Part model, mm, in its own coordinate system. A direction names the side the tool comes from. Give positions to 0.01 mm unless a question says otherwise; leave off trailing zeros. Order: outer loops, then holes, each group sorted by start corner. A loop starts at its lowest first (then second) coordinate and runs counter-clockwise, first axis right, second up. Notation, with made-up numbers: M 15,-21 L 57,-21 A19 cw 57,-12 Z; hole C 44.5,58.25 d6. An arc over 180 degrees is marked long. Answer as a JSON object with one key per item and string values.
from build123d import *

# Parameters (mm, degrees)
SKETCH1_W           = 190.5
SKETCH1_H           = 76.2
BOSS_EXTRUDE1_DEPTH = 6.35
SKETCH2_W           = 6.35
SKETCH2_H           = 50.8
BOSS_EXTRUDE2_DEPTH = 6.35
SKETCH3_W           = 6.35
SKETCH3_H           = 50.8
BOSS_EXTRUDE3_DEPTH = 6.35
SKETCH4_W           = 38.1
SKETCH4_H           = 6.35
BOSS_EXTRUDE4_DEPTH = 6.35
SKETCH6_R           = 1.524
CUT_EXTRUDE4_DEPTH  = 6.35


with BuildPart() as part:
    # Sketch1 → Boss-Extrude1 (new body)
    with BuildSketch(Plane.XY):
        Rectangle(SKETCH1_W, SKETCH1_H)
    extrude(amount=BOSS_EXTRUDE1_DEPTH)

    # Sketch2 → Boss-Extrude2 (add)
    with BuildSketch(Plane.ZY.offset(95.25)):
        with Locations((3.175, 0)):
            Rectangle(SKETCH2_W, SKETCH2_H)
    extrude(amount=BOSS_EXTRUDE2_DEPTH)

    # Sketch3 → Boss-Extrude3 (add)
    with BuildSketch(Plane(origin=(95.25, 0, 0), x_dir=(0, 0, -1), z_dir=(1, 0, 0))):
        with Locations((-3.175, 0)):
            Rectangle(SKETCH3_W, SKETCH3_H)
    extrude(amount=BOSS_EXTRUDE3_DEPTH)

    # Sketch4 → Boss-Extrude4 (add)
    with BuildSketch(Plane.XZ.offset(38.1)):
        with Locations((-50.8, 3.175)):
            Rectangle(SKETCH4_W, SKETCH4_H)
        with Locations((50.8, 3.175)):
            Rectangle(SKETCH4_W, SKETCH4_H)
    extrude(amount=BOSS_EXTRUDE4_DEPTH)

    # Sketch6 → Cut-Extrude4 (cut)
    with BuildSketch(Plane(origin=(23.763692911, 98.5857123, 0), x_dir=(-1, 0, 0), z_dir=(0, 0, -1))):
        with Locations((-61.961307089, -120.8107123)):
            Circle(SKETCH6_R)
        with Locations((109.488692911, -120.8107123)):
            Circle(SKETCH6_R)
    extrude(amount=-CUT_EXTRUDE4_DEPTH, mode=Mode.SUBTRACT)


solid = part.part
1. Two-plate mould, pull along X, no slides. Class faces 6 (the flat face through (31.75, -41, 3)), 7 (the flat face through (95.25, 32, 3)), 8 (the flat face through (-1, 38.1, 3)): +X half, -X half, draft (parallel to the pull), parting line (faces both ways), or undercut.
Worked answers:
{"face 6": "undercut", "face 7": "+X half", "face 8": "draft"}
2. Cut at B-B on x = -21.5. Give the cut face in (y, z).
Worked answers:
{"outline": "M -38.1,0 L 38.1,0 L 38.1,6.35 L -38.1,6.35 Z"}
3. Which spindle directions (+Z, -Z, +X, -X, +Y, -Y) get a long thin tool onto all of the face, cutting with end or side? Do faces 1 (the flat face through (-95.25, -32, 3)), 2 (the flat face through (98, -25.4, 3)), 3 (the flat face through (98, 25.4, 3)), 4 (the flat face through (-95.25, 32, 3)), 5 (the flat face through (101.6, 0, 3)). Say none if no direction does.
Worked answers:
{"face 1": "+Z, -Z, -X, -Y", "face 2": "+Z, -Z, +X, -Y", "face 3": "+Z, -Z, +X, +Y", "face 4": "+Z, -Z, -X, +Y", "face 5": "+Z, -Z, +X, +Y, -Y"}
4. Pin check, flat tips, straight feed: P1, Ø12, axis at x = 69.5, y = -17, coming from the -Z side; P2, Ø3, axis at y = -34, z = 3, coming from the -X side; P3, Ø3, axis at x = -6.5, z = 3, coming from the -Y side; P4, Ø3, axis at y = -43, z = 3.5, coming from the +X side. Stop position of each tip, or through.
Worked answers:
{"P1": "stops at z = 0", "P2": "stops at x = -95.25", "P3": "stops at y = -38.1", "P4": "stops at x = 69.85"}
5. Cut at A-A on z = 2.25. Give the cut face in (x, y) (3 decimals), plus the area to 3 significant figures.
Worked answers:
{"outline": "M -101.6,-25.4 L -95.25,-25.4 L -95.25,-38.1 L -69.85,-38.1 L -69.85,-44.45 L -31.75,-44.45 L -31.75,-38.1 L 31.75,-38.1 L 31.75,-44.45 L 69.85,-44.45 L 69.85,-38.1 L 95.25,-38.1 L 95.25,-25.4 L 101.6,-25.4 L 101.6,25.4 L 95.25,25.4 L 95.25,38.1 L -95.25,38.1 L -95.25,25.4 L -101.6,25.4 Z; hole C -85.725,-22.225 d3.048; hole C 85.725,-22.225 d3.048", "area": "15,600 mm^2"}
6. Cut at C-C on y = -32. Give the cut face in (x, z).
Worked answers:
{"outline": "M -95.25,0 L 95.25,0 L 95.25,6.35 L -95.25,6.35 Z"}
7. Probe line 1 along X through (y, z) = (-41, 3); line 2 along X through (y, z) = (30, 4); line 3 along Y through (x, z) = (-85.5, 1.5). List the from-to ranges inside material, lowest first.
Worked answers:
{"line 1": "x = -69.85 to -31.75, 31.75 to 69.85", "line 2": "x = -95.25 to 95.25", "line 3": "y = -38.1 to -23.73, -20.72 to 38.1"}
